from build123d import *

# Parameters (mm, degrees)
SKETCH3_R          = 2.25
CUT_EXTRUDE1_DEPTH = 5


with BuildPart() as part:
    # Sketch2 → Revolve1 (revolve)
    with BuildSketch(Plane(origin=(0, 0, 0), x_dir=(1, 0, 0), z_dir=(0, 1, 0))):
        Polygon((5, -17.47), (5, 9.73), (15, 9.73), (15, 2.3), (23.75, 2.3), (23.75, 0), (15, 0), (15, -17.47), align=None)
    revolve(axis=Axis((0, 0, 39.284955752), (0, 0, -1)))

    # Sketch3 → Cut-Extrude1 (cut, symmetric)
    with BuildSketch(Plane.XY):
        with Locations((0, 20.25)):
            Circle(SKETCH3_R)
        with Locations((17.537014427, -10.125)):
            Circle(SKETCH3_R)
        with Locations((-17.537014427, -10.125)):
            Circle(SKETCH3_R)
    extrude(amount=CUT_EXTRUDE1_DEPTH, both=True, mode=Mode.SUBTRACT)


solid = part.part
Design review of the part built by this model. Coordinates are the model's own, in mm. A direction names the side the tool comes from. Round coordinates to 2 decimals unless told otherwise and drop trailing zeros. Write each loop counter-clockwise with the first axis right and the second up, starting at its lowest first coordinate (ties: lowest second). Pieces come first, ordered by that corner, then holes.
Item 1: Consider section C-C on z = 10.25. Give the boundary of the cut face in (x, y).
Item 2: Draft analysis for pull direction Y (two halves, no side actions). For faces 1 (the flat face through (4, -4, -9.73)), 2 (the cylindrical face through (-19.195, -8.604, -1.134)), 3 (the cylindrical face through (-5.149, 23.185, -1.134)), state which applies: released by +Y, released by -Y, zero draft, split by the parting line, or undercut.
Item 3: Wall thickness on L1, parallel to Y at x = 0, z = 12.25; L2, parallel to Z at x = 15, y = -15: over which ranges is each line inside the solid? List them lowest first.
Item 4: Consider section B-B on x = -17. Give the boundary of the cut face in (y, z) (3 decimals).
Item 5: Consider section A-A on y = 0. Give the boundary of the cut face in (x, z), and give its area (3 significant figures).
Item 6: Consider section D-D on x = 6. Give the boundary of the cut face in (y, z).
Item 7: For pin 1 Ø1 at (y, z) = (-10, 5.5) entering from +X; pin 2 Ø4 at (y, z) = (-13, -1) entering from +X; pin 3 Ø7 at (x, y) = (17.54, -10.12) entering from -Z, all flat-tipped, find the tip position at first contact; note any pin that passes through.
Item 8: For faces 4 (the flat face through (16, 0, 0)), 5 (the flat face through (-16, 0, -2.3)), 6 (the cylindrical face through (18.7, -8.2, -1.1)), list the 3-axis set-ups (+Z, -Z, +X, -X, +Y, -Y) from which the entire face can be reached by the end or side of a thin tool; tool diameter is ignored.
Check values:
1. outline: circle Ø30 at (0, 0); hole circle Ø10 at (0, 0)
2. face 1: zero draft
2. face 2: undercut
2. face 3: split by the parting line
3. L1: y = -15 to -5, 5 to 15
3. L2: z = -2.3 to 0
4. outline: (-16.585, -2.3) - (-12.31, -2.3) - (-12.31, 0) - (-16.585, 0) - close; (-7.94, -2.3) - (16.585, -2.3) - (16.585, 0) - (-7.94, 0) - close
5. outline: (-23.75, -2.3) - (-15, -2.3) - (-15, -9.73) - (-5, -9.73) - (-5, 17.47) - (-15, 17.47) - (-15, 0) - (-23.75, 0) - close; (5, -9.73) - (15, -9.73) - (15, -2.3) - (23.75, -2.3) - (23.75, 0) - (15, 0) - (15, 17.47) - (5, 17.47) - close
5. area: 584 mm2
6. outline: (-22.98, -2.3) - (-13.75, -2.3) - (-13.75, -9.73) - (13.75, -9.73) - (13.75, -2.3) - (22.98, -2.3) - (22.98, 0) - (13.75, 0) - (13.75, 17.47) - (-13.75, 17.47) - (-13.75, 0) - (-22.98, 0) - close
7. pin 1: stops at x = 11.61
7. pin 2: stops at x = 21.05
7. pin 3: stops at z = -2.3
8. face 4: +Z
8. face 5: -Z
8. face 6: +Z, -Z
